Part model, mm, in its own coordinate system. A direction names the side the tool comes from. Round coordinates to 2 decimals unless told otherwise and drop trailing zeros. Write each loop counter-clockwise with the first axis right and the second up, starting at its lowest first coordinate (ties: lowest second). Pieces come first, ordered by that corner, then holes.
1) Which spindle directions (+Z, -Z, +X, -X, +Y, -Y) get a long thin tool onto all of the face, cutting with end or side? Do faces 1 (the cylindrical face through (-11.361, -18.605, 31.186)), 2 (the flat face through (-16.3, 5.7, 32.2)). Say none if no direction does.
2) Saw through at C-C on z = 34. Write the cut outline in (x, y), and give its area (3 significant figures).
3) Saw through at B-B on x = 0. Write the cut outline in (y, z), and give its area (3 significant figures).
4) Saw through at A-A on y = 0. Write the cut outline in (x, z).
5) Drill centre lines: L1, parallel to Y at x = -10.25, z = 31.6; L2, parallel to Y at x = 0, z = 34.5; L3, parallel to Z at x = 6.5, y = -18.5. Where is each one in solid material? Low to high.
6) Pull direction Y, two halves, no side cores. Call faces 3 (the cylindrical face through (21.79, -0.54, 31.19)), 4 (the cylindrical face through (-23.977, 1.055, 31.186)), 5 (the flat face through (4, -4, 36.2)): +Y half, -Y half, draft (parallel to the pull), parting line (faces both ways), or undercut.
7) Saw through at D-D on x = -10.25. Write the cut outline in (y, z).
8) Flat gauge pins, fed straight in: pin 1 (1 mm diameter, centred on y = 13.5, z = 35.5, fed in from +X); pin 2 (2 mm diameter, centred on x = -10.25, y = 17.75, fed in from +Z); pin 3 (1.5 mm diameter, centred on y = 13.5, z = 33.5, fed in from -X). Where does each tip first touch, or does it go through?
```python
from build123d import *

# Parameters (mm, degrees)
CYLINDER058_R     = 1.4
CYLINDER058_DEPTH = 2
ARRAY012_COUNT    = 3
CYLINDER057_R     = 4.9
CYLINDER057_DEPTH = 6
CYLINDER056_R     = 24
CYLINDER056_DEPTH = 2
CYLINDER055_R     = 17
CYLINDER055_DEPTH = 4


with BuildPart() as screw_holes:
    # Cylinder058 → Cylinder058 (new body)
    with BuildSketch(Plane(origin=(20.5, 0, 0), x_dir=(1, 0, 0), z_dir=(0, 0, 1))):
        Circle(CYLINDER058_R)
    extrude(amount=CYLINDER058_DEPTH)

    # Array012: screw-holes ×3 about axis
    array012_axis = Axis((0, 0, 0), (0, 0, 1))


with BuildPart() as screw_holes_1:
    add(screw_holes.part)
    for i in range(1, ARRAY012_COUNT):
        add(screw_holes.part.rotate(array012_axis, i * 360 / ARRAY012_COUNT))


with BuildPart() as pot_thread_hole:
    # Cylinder057 → Cylinder057 (new body)
    with BuildSketch(Plane.XY):
        Circle(CYLINDER057_R)
    extrude(amount=CYLINDER057_DEPTH)


with BuildPart() as brim:
    # Cylinder056 → Cylinder056 (new body)
    with BuildSketch(Plane.XY):
        Circle(CYLINDER056_R)
    extrude(amount=CYLINDER056_DEPTH)


with BuildPart() as pot_mount001:
    # Cylinder055 → Cylinder055 (new body)
    with BuildSketch(Plane.XY.offset(2)):
        Circle(CYLINDER055_R)
    extrude(amount=CYLINDER055_DEPTH)

    # Fusion025: union brim
    add(brim.part)

    # Cut046: cut pot-thread-hole
    add(pot_thread_hole.part, mode=Mode.SUBTRACT)

    # Cut047: cut screw-holes
    add(screw_holes_1.part, mode=Mode.SUBTRACT)


with BuildPart() as pot_mount001_1:
    # Cut047 placement: moved
    add(pot_mount001.part.moved(Location((0, 0, 30.2))))


solid = pot_mount001_1.part
```
Completed:
1. face 1: +Z, -Z
1. face 2: +Z
2. outline: circle Ø34 at (0, 0); hole circle Ø9.8 at (0, 0)
2. area: 832 mm2
3. outline: (-24, 30.2) - (-4.9, 30.2) - (-4.9, 36.2) - (-17, 36.2) - (-17, 32.2) - (-24, 32.2) - close; (4.9, 30.2) - (24, 30.2) - (24, 32.2) - (17, 32.2) - (17, 36.2) - (4.9, 36.2) - close
3. area: 173 mm2
4. outline: (-24, 30.2) - (-4.9, 30.2) - (-4.9, 36.2) - (-17, 36.2) - (-17, 32.2) - (-24, 32.2) - close; (4.9, 30.2) - (19.1, 30.2) - (19.1, 32.2) - (17, 32.2) - (17, 36.2) - (4.9, 36.2) - close; (21.9, 30.2) - (24, 30.2) - (24, 32.2) - (21.9, 32.2) - close
5. L1: y = -21.7 to -19.15, -16.35 to 16.35, 19.15 to 21.7
5. L2: y = -17 to -4.9, 4.9 to 17
5. L3: z = 30.2 to 32.2
6. face 3: undercut
6. face 4: parting line
6. face 5: draft
7. outline: (-21.7, 30.2) - (-19.15, 30.2) - (-19.15, 32.2) - (-21.7, 32.2) - close; (-16.35, 30.2) - (16.35, 30.2) - (16.35, 32.2) - (13.56, 32.2) - (13.56, 36.2) - (-13.56, 36.2) - (-13.56, 32.2) - (-16.35, 32.2) - close; (19.15, 30.2) - (21.7, 30.2) - (21.7, 32.2) - (19.15, 32.2) - close
8. pin 1: stops at x = 10.95
8. pin 2: passes through
8. pin 3: stops at x = -11.24
